Part model, mm, in its own coordinate system. Give positions to 0.01 mm unless a question says otherwise; leave off trailing zeros. Order: outer loops, then holes, each group sorted by start corner. A loop starts at its lowest first (then second) coordinate and runs counter-clockwise, first axis right, second up. Notation, with made-up numbers: M 84.25,18 L 118.25,18 A23 cw 118.25,48 Z; hole C 46,56.25 d7. An arc over 180 degrees is marked long. Answer as a JSON object with one key per item and string values.
from build123d import *

# Parameters (mm, degrees)
SKETCH1_W           = 160
SKETCH1_H           = 272
SKETCH1_R           = 1.75
BOSS_EXTRUDE1_DEPTH = 10
SKETCH3_R           = 3
CUT_EXTRUDE1_DEPTH  = 18


with BuildPart() as part:
    # Sketch1 → Boss-Extrude1 (new body)
    with BuildSketch(Plane(origin=(0, 0, 0), x_dir=(1, 0, 0), z_dir=(0, 1, 0))):
        with Locations((80, 136)):
            Rectangle(SKETCH1_W, SKETCH1_H)
        with Locations(Location((4.328403696, 232, 0), (0, 0, 270))):
            Circle(SKETCH1_R, mode=Mode.SUBTRACT)
        with Locations(Location((4.328403696, 252, 0), (0, 0, 270))):
            Circle(SKETCH1_R, mode=Mode.SUBTRACT)
        with Locations(Location((4.328403696, 40, 0), (0, 0, 90))):
            Circle(SKETCH1_R, mode=Mode.SUBTRACT)
        with Locations(Location((4.328403696, 20, 0), (0, 0, 90))):
            Circle(SKETCH1_R, mode=Mode.SUBTRACT)
        with Locations(Location((155.671596304, 20, 0), (0, 0, 270))):
            Circle(SKETCH1_R, mode=Mode.SUBTRACT)
        with Locations(Location((155.671596304, 40, 0), (0, 0, 270))):
            Circle(SKETCH1_R, mode=Mode.SUBTRACT)
        with Locations(Location((155.671596304, 232, 0), (0, 0, 90))):
            Circle(SKETCH1_R, mode=Mode.SUBTRACT)
        with Locations(Location((155.671596304, 252, 0), (0, 0, 90))):
            Circle(SKETCH1_R, mode=Mode.SUBTRACT)
    extrude(amount=BOSS_EXTRUDE1_DEPTH)

    # Sketch3 → Cut-Extrude1 (cut)
    with BuildSketch(Plane(origin=(0, 10, 0), x_dir=(1, 0, 0), z_dir=(0, 1, 0))):
        with Locations(Location((108, 134, 0), (0, 0, 270))):
            Circle(SKETCH3_R)
        with Locations(Location((108, 215, 0), (0, 0, 270))):
            Circle(SKETCH3_R)
    extrude(amount=-CUT_EXTRUDE1_DEPTH, mode=Mode.SUBTRACT)


solid = part.part
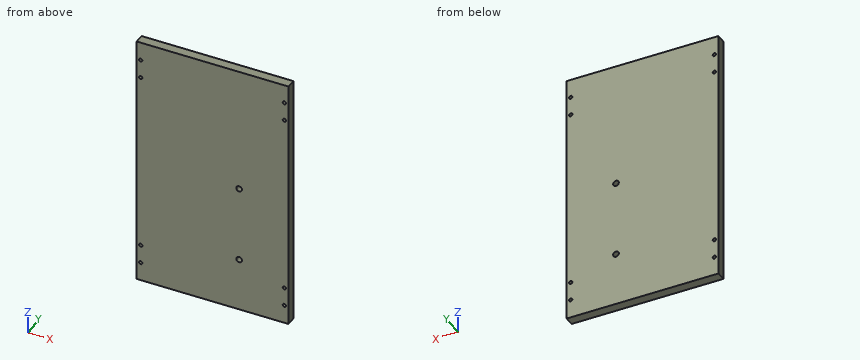
1. Cut at B-B on z = -134. Give the cut face in (x, y).
Worked answers:
{"outline": "M 0,0 L 105,0 L 105,10 L 0,10 Z; M 111,0 L 160,0 L 160,10 L 111,10 Z"}
2. Probe line 1 along X through (y, z) = (7, -20); line 2 along X through (y, z) = (3.75, -134); line 3 along X through (y, z) = (7.25, -233.5). List the from-to ranges inside material, lowest first.
Worked answers:
{"line 1": "x = 0 to 2.58, 6.08 to 153.92, 157.42 to 160", "line 2": "x = 0 to 105, 111 to 160", "line 3": "x = 0 to 3.43, 5.23 to 154.77, 156.57 to 160"}
3. Cut at A-A on x = 108. Give the cut face in (y, z), plus the area to 3 significant figures.
Worked answers:
{"outline": "M 0,-272 L 10,-272 L 10,-218 L 0,-218 Z; M 0,-212 L 10,-212 L 10,-137 L 0,-137 Z; M 0,-131 L 10,-131 L 10,0 L 0,0 Z", "area": "2,600 mm^2"}
